from build123d import *

# Parameters (mm, degrees)
ESBO_O1_W                = 20
ESBO_O1_H                = 28
ESBO_O1_R                = 1.5
RESSALTO_EXTRUS_O1_DEPTH = 6
ESBO_O2_W                = 5
ESBO_O2_H                = 12
RESSALTO_EXTRUS_O2_START = -33
ESBO_O3_W                = 20
ESBO_O3_H                = 20
RESSALTO_EXTRUS_O2_DEPTH = 10
CORTE_EXTRUS_O1_DEPTH    = 28


with BuildPart() as part:
    # Esboço1 → Ressalto-extrusão1 (new body, symmetric)
    with BuildSketch(Plane.XY):
        Rectangle(ESBO_O1_W, ESBO_O1_H)
        with Locations((-7, 10)):
            Circle(ESBO_O1_R, mode=Mode.SUBTRACT)
        with Locations((7, 10)):
            Circle(ESBO_O1_R, mode=Mode.SUBTRACT)
    extrude(amount=RESSALTO_EXTRUS_O1_DEPTH, both=True)

    # Esboço2 → Revolução1 (revolve)
    with BuildSketch(Plane.XY):
        Polygon((3, -33), (3, -23), (3, -14), (0, -14), (0, -38), (0.75, -38), (3.5, -36), (3.5, -33), align=None)
        with Locations((2.5, 20)):
            Rectangle(ESBO_O2_W, ESBO_O2_H)
    revolve(axis=Axis((0, 0, 0), (0, -1, 0)))

    # Esboço3 → Ressalto-extrusão2 (add)
    with BuildSketch(Plane(origin=(0, 0, 0), x_dir=(1, 0, 0), z_dir=(0, 1, 0)).offset(RESSALTO_EXTRUS_O2_START)):
        with Locations((0, 4)):
            Rectangle(ESBO_O3_W, ESBO_O3_H)
    extrude(amount=RESSALTO_EXTRUS_O2_DEPTH)

    # Esboço4 → Corte-extrusão1 (cut)
    with BuildSketch(Plane(origin=(0, 14, 0), x_dir=(1, 0, 0), z_dir=(0, 1, 0))):
        with BuildLine():
            ThreePointArc((-10, 0), (-9.486832981, 3.16227766), (-8, 6))
            Line((-8, 6), (-10, 6))
            Line((-10, 6), (-10, 0))
        make_face()
        with BuildLine():
            ThreePointArc((-8, -6), (-9.486832981, -3.16227766), (-10, 0))
            Line((-10, 0), (-10, -6))
            Line((-10, -6), (-8, -6))
        make_face()
        with BuildLine():
            Line((10, -6), (10, 0))
            ThreePointArc((10, 0), (9.486832981, -3.16227766), (8, -6))
            Line((8, -6), (10, -6))
        make_face()
        with BuildLine():
            Line((10, 6), (8, 6))
            ThreePointArc((8, 6), (9.486832981, 3.16227766), (10, 0))
            Line((10, 0), (10, 6))
        make_face()
    extrude(amount=-CORTE_EXTRUS_O1_DEPTH, mode=Mode.SUBTRACT)


solid = part.part
Input: part model. Units: mm. Frame: model coordinates. A direction names the side the tool comes from. Give positions to 0.01 mm unless a question says otherwise; leave off trailing zeros. Order: outer loops, then holes, each group sorted by start corner. A loop starts at its lowest first (then second) coordinate and runs counter-clockwise, first axis right, second up. Notation, with made-up numbers: M 66.5,30 L 81.5,30 A27 ccw 81.5,59 Z; hole C 5,-26.5 d4. An arc over 180 degrees is marked long. Answer as a JSON object with one key per item and string values.
1. Pull-direction query (X, two-part tool) for faces 1 (the conical face through (0.5, -37.87, 0.78)), 2 (the cylindrical face through (-5.614, 9.425, -0.084)), 3 (the flat face through (0, 0, 6)); classes: +X half, -X half, draft (parallel to the pull), parting line (faces both ways), or undercut.
Result sheet:
{"face 1": "parting line", "face 2": "undercut", "face 3": "draft"}
2. Cut plane C-C, the plane y = 10. Output: boundary loops of the cut face in (x, z), and give its area (3 significant figures).
Result sheet:
{"outline": "M -8.5,-5.27 L -8.5,5.27 A10 ccw Z; M -5.5,-6 L 5.5,-6 L 5.5,6 L -5.5,6 Z; M 8.5,-5.27 A10 ccw 8.5,5.27 Z", "area": "153 mm²"}
3. Cut plane B-B, the plane x = 7. Output: boundary loops of the cut face in (y, z).
Result sheet:
{"outline": "M -33,-14 L -23,-14 L -23,6 L -33,6 Z; M -14,-6 L 8.5,-6 L 8.5,6 L -14,6 Z; M 11.5,-6 L 14,-6 L 14,6 L 11.5,6 Z"}
4. Ray query, line 1 (Y direction, x = 7, z = -2.75); line 2 (Y direction, x = 3, z = -5.25); line 3 (Y direction, x = 5.25, z = -10). Return the intervals inside material, ascending. Write a range as [from, to].
Result sheet:
{"line 1": "[-33, -23], [-14, 8.5], [11.5, 14]", "line 2": "[-33, -23], [-14, 14]", "line 3": "[-33, -23]"}
5. Reachability of faces 4 (the cylindrical face through (3.233, -34.479, -1.341)), 5 (the flat face through (10, -28, -4)), 6 (the cylindrical face through (-1.08, 20.08, -4.88)), 7 (the flat face through (0, 0, -6)), 8 (the flat face through (-2, -14, -3)) from +Z, -Z, +X, -X, +Y, -Y: full face, straight path, thin tool, end or side. Return the list, or none.
Result sheet:
{"face 4": "-Y", "face 5": "+Z, -Z, +X, +Y, -Y", "face 6": "+Y", "face 7": "-Z, +X, -X, +Y", "face 8": "none"}
6. Cut plane D-D, the plane x = 0. Output: boundary loops of the cut face in (y, z), and give its area (4 significant figures).
Result sheet:
{"outline": "M -38,-0.75 L -36,-3.5 L -33,-3.5 L -33,-14 L -23,-14 L -23,-3 L -14,-3 L -14,-6 L 14,-6 L 14,-5 L 26,-5 L 26,5 L 14,5 L 14,6 L -14,6 L -14,3 L -23,3 L -23,6 L -33,6 L -33,3.5 L -36,3.5 L -38,0.75 Z", "area": "739.5 mm²"}
7. Cut plane A-A, the plane z = 4.25. Output: boundary loops of the cut face in (x, y).
Result sheet:
{"outline": "M -10,-33 L 10,-33 L 10,-23 L -10,-23 Z; M -9.05,-14 L 9.05,-14 L 9.05,14 L 2.63,14 L 2.63,26 L -2.63,26 L -2.63,14 L -9.05,14 Z; hole C -7,10 d3; hole C 7,10 d3"}
8. First-contact query: P1, Ø3, axis at x = 2, z = -8, coming from the +Y side; P2, Ø8, axis at x = -2.5, y = -1.5, coming from the -Z side; P3, Ø8, axis at x = -4, z = -5.5, coming from the -Y side. Flat tips, straight axial feed; report the tip coordinate or a pass-through.
Result sheet:
{"P1": "y = -23", "P2": "z = -6", "P3": "y = -36.51"}
